```python
from build123d import *

# Parameters (mm, degrees)
F0_R     = 1.5
F1_DEPTH = 3.175
F3_DEPTH = 12.5


with BuildPart() as f1:
    # F0 (on Top) → F1 (new body)
    with BuildSketch(Plane.XY):
        with BuildLine():
            Line((0, 38.1), (0, 44.323))
            Line((0, 44.323), (-33.461, 44.323))
            ThreePointArc((-33.461, 44.323), (-38.9926963492, 42.0316963492), (-41.284, 36.5))
            Line((-41.284, 36.5), (-41.284, 7.823))
            ThreePointArc((-41.284, 7.823), (-43.5753036508, 2.2913036508), (-49.107, 0))
            Line((-49.107, 0), (-73.882, 0))
            ThreePointArc((-73.882, 0), (-75.0494332957, -0.4835667043), (-75.533, -1.651))
            Line((-75.533, -1.651), (-75.533, -27.813))
            ThreePointArc((-75.533, -27.813), (-75.0494332957, -28.9804332957), (-73.882, -29.464))
            Line((-73.882, -29.464), (0, -29.464))
            Line((0, -29.464), (0, 0))
            Line((0, 0), (-10.232, 0))
            add(Edge.make_bspline(
                [(-10.232, 38.1), (-35.632, 38.1), (-35.632, 19.05), (-35.632, 0), (-10.232, 0)],
                knots=[1.5707963268, 1.5707963268, 1.5707963268, 3.1415926536, 3.1415926536, 4.7123889804, 4.7123889804, 4.7123889804], degree=2, weights=[1, 0.7071067812, 1, 0.7071067812, 1]))
            Line((-10.232, 38.1), (0, 38.1))
        make_face()
        with Locations((-70.042, -22.232)):
            Circle(F0_R, mode=Mode.SUBTRACT)
        with Locations((-57.042, -22.232)):
            Circle(F0_R, mode=Mode.SUBTRACT)
        with Locations((-70.042, -11.232)):
            Circle(F0_R, mode=Mode.SUBTRACT)
        with Locations((-57.042, -11.232)):
            Circle(F0_R, mode=Mode.SUBTRACT)
    extrude(amount=F1_DEPTH)

    # F2 (on Top) → F3 (cut, symmetric)
    with BuildSketch(Plane.XY):
        with BuildLine():
            Line((-20.6375, 50.55129749), (-20.6375, 40.513))
            ThreePointArc((-20.6375, 40.513), (-19.05, 38.9255), (-17.4625, 40.513))
            Line((-17.4625, 40.513), (-17.4625, 50.55129749))
            Line((-17.4625, 50.55129749), (-20.6375, 50.55129749))
        make_face()
        with BuildLine():
            Line((-17.4625, 7.62629749), (-20.6375, 7.62629749))
            Line((-20.6375, 7.62629749), (-20.6375, -2.412))
            ThreePointArc((-20.6375, -2.412), (-19.05, -3.9995), (-17.4625, -2.412))
            Line((-17.4625, -2.412), (-17.4625, 7.62629749))
        make_face()
    extrude(amount=F3_DEPTH, both=True, mode=Mode.SUBTRACT)

    # F4: F1 across plane


with BuildPart() as f1_1:
    add(f1.part)
    add(f1.part.mirror(Plane.YZ))


solid = f1_1.part
```
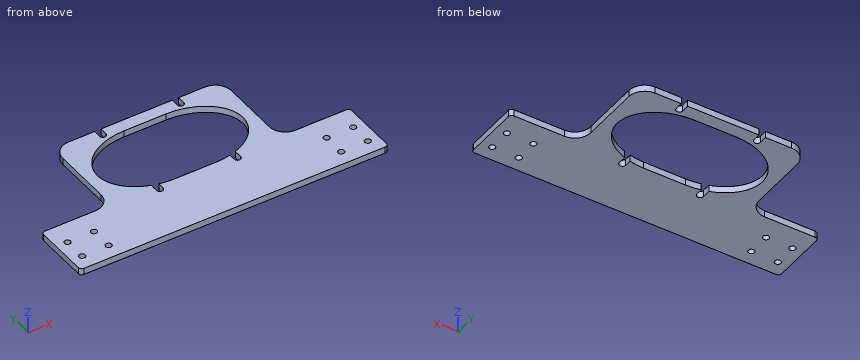
Can you work these out from the model? Positions are in its coordinate system, mm. Coordinates: 2 decimals unless noted, no trailing zeros. Put each result on its own line as item: value. Start each with the question number.
Q1. I'm going to push flat-ended pins straight in: P1, Ø2.5, axis at x = 57.042, y = -11.232, coming from the -Z side; P2, Ø1.6, axis at y = 0, z = 2.5, coming from the -X side; P3, Ø1, axis at y = 43, z = 1.5, coming from the -X side; P4, Ø1, axis at x = -65.5, z = 1.5, coming from the +Y side. Where does each tip first touch, or does it pass through?
Q2. I want a section at A-A (z = 0.75). Count the separate pieces of the cut face and the enclosed holes in it, plus the area to 3 significant figures.
Q3. If I drill on line 1 (Y direction, x = -6.5, z = 1.6); line 2 (X direction, y = 19, z = 0.85); line 3 (X direction, y = 14, z = 3), over which ranges is the centre line in solid material (lowest first)? Write a range as [from, to].
Taken from the geometry:
1. P1: passes through
1. P2: stops at x = -75.3
1. P3: stops at x = -38.48
1. P4: stops at y = 0
2. separate pieces: 1
2. enclosed holes: 9
2. area: 5,690 mm2
3. line 1: y = [-29.46, 0], [38.1, 44.32]
3. line 2: x = [-41.28, -35.63], [35.63, 41.28]
3. line 3: x = [-41.28, -34.72], [34.72, 41.28]
